```python
from build123d import *

# Parameters (mm, degrees)
BOSS_EXTRUDE1_DEPTH = 40
FILLET1_R           = 0.5


with BuildPart() as part:
    # Sketch1 → Boss-Extrude1 (new body)
    with BuildSketch(Plane(origin=(0, 0, 0), x_dir=(-1, 0, 0), z_dir=(0, 1, 0))):
        Polygon((22.228552834, -5.26e-07), (0, -25.478873765), (-22.228552834, -5.26e-07), (0, 25.478872714), align=None)
    extrude(amount=BOSS_EXTRUDE1_DEPTH)

    # Fillet1
    fillet1_edges = [part.edges().sort_by_distance(p)[0] for p in [
        (11.114276417, 40, -12.739437146),
        (-11.114276417, 40, -12.739437146),
        (-11.114276417, 40, 12.739436094),
        (-11.114276417, 0, -12.739437146),
        (11.114276417, 0, -12.739437146),
        (11.114276417, 0, 12.739436094),
        (-11.114276417, 0, 12.739436094),
        (11.114276417, 40, 12.739436094),
    ]]
    fillet(fillet1_edges, radius=FILLET1_R)


solid = part.part
```
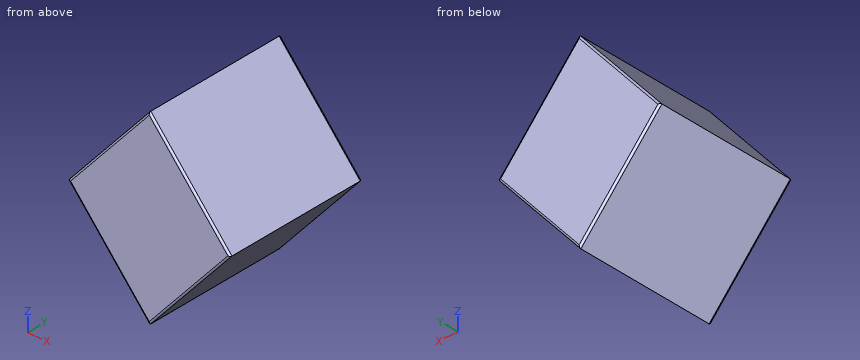
Design review of the part built by this model. Coordinates are the model's own, in mm. Coordinates: 2 decimals unless noted, no trailing zeros. Loops run counter-clockwise (first coordinate to the right, second up) from the corner with the lowest first, then second, coordinate; pieces in that order, holes last.
Q1. To check wall thickness, follow line 1 (Z direction, x = 2.5, y = 37.5); line 2 (X direction, y = 35, z = -8); line 3 (Z direction, x = -2, y = 22). State the ranges of each line that lie inside material, in increasing order.
Reported:
line 1: z = -22.61 to 22.61
line 2: x = -15.25 to 15.25
line 3: z = -23.19 to 23.19
Q2. For pin 1 (10 mm diameter, centred on x = -7, y = 21.5, fed in from +Z); pin 2 (1.5 mm diameter, centred on x = -15.5, y = 11.5, fed in from -Z); pin 3 (10 mm diameter, centred on y = 35.5, z = -15.5, fed in from +X), all flat-tipped, find the tip position at first contact; note any pin that passes through.
Reported:
pin 1: stops at z = 23.19
pin 2: stops at z = -8.57
pin 3: stops at x = 13.07
Q3. We need section A-A on y = 29. State the section outline as (x, z) points.
Reported:
outline: (-22.23, 0) - (0, -25.48) - (22.23, 0) - (0, 25.48) - close
